For this review, take the finished solid that the model builds, in its own axes (mm). A direction names the side the tool comes from. Round coordinates to 2 decimals unless told otherwise and drop trailing zeros. Write each loop counter-clockwise with the first axis right and the second up, starting at its lowest first coordinate (ties: lowest second). Pieces come first, ordered by that corner, then holes. Notation, with made-up numbers: (7.5, 48) -> (51.5, 48) arc R8 ccw to (51.5, 53) -> close; hole circle Ø3 at (24.5, 17). An arc over 180 degrees is marked (long way). Write each question's results on one line, items separated by ' | '. Start each with the question number.
Item 1: Add section C-C (x = 33.65). State the section outline as (y, z) points, plus the area to 3 significant figures.
Item 2: Clearance check with flat-ended pins moving along their axes: pin 1 (8 mm diameter, centred on x = 13.25, y = -55.25, fed in from -Z); pin 2 (3 mm diameter, centred on y = -66, z = -5.5, fed in from +X); pin 3 (5 mm diameter, centred on x = 13, z = -3.5, fed in from +Y). State where each tip first meets the part, or that it passes through.
Item 3: Add section A-A (y = -38). State the section outline as (x, z) points, plus the area to 3 significant figures.
Item 4: Tool access review of faces 1 (the flat face through (11, -41, 1.2)), 2 (the cylindrical face through (-31.49, -19.65, 0.59)): name each direction out of +Z, -Z, +X, -X, +Y, -Y from which nothing blocks a thin tool from reaching the whole face with its end or side.
Item 5: Add section B-B (x = -39.75). State the section outline as (y, z) points.
Item 6: Add section D-D (z = -4.5). State the section outline as (x, y) points.
Item 7: The part is to be moulded in two halves that separate along X. For faces 3 (the cylindrical face through (-39.01, -43.17, 0.59)), 4 (the flat face through (14.5, -67, -5)), 5 (the flat face through (8.5, -67, -5)), say which applies: +X half, -X half, draft (parallel to the pull), parting line (faces both ways), or undercut.
Item 8: To check wall thickness, follow line 1 along Y through (x, z) = (-23.55, 0.7) (3 decimals); line 2 along Y through (x, z) = (2.75, 0.6); line 3 along X through (y, z) = (-58.5, 0.75). State the ranges of each line that lie inside material, in increasing order.
from build123d import *

# Parameters (mm, degrees)
SKETCH1_W                                    = 109.5
SKETCH1_H                                    = 82.5
SKETCH1_R                                    = 1.6
SKETCH1_R_2                                  = 1.05
SKETCH1_R_3                                  = 1.75
BOSS_EXTRUDE1_DEPTH                          = 1.2
CSK_FOR_M3_FLAT_COUNTERSUNK_HEAD_SCR_2_COUNT = 2
CSK_FOR_M3_FLAT_COUNTERSUNK_HEAD_SCR_2_PITCH = 76
CSK_FOR_M3_FLAT_COUNTERSUNK_HEAD_SCR_3_COUNT = 2
CSK_FOR_M3_FLAT_COUNTERSUNK_HEAD_SCR_3_PITCH = 122.834237898
CSK_FOR_M3_FLAT_COUNTERSUNK_HEAD_SCR_4_COUNT = 2
CSK_FOR_M3_FLAT_COUNTERSUNK_HEAD_SCR_4_PITCH = 96.5
F_2_6_2_6_DIAMETER_HOLE1_D                   = 2.6
CUT_EXTRUDE1_REACH                           = 101.438
SKETCH9_R                                    = 1.05
SKETCH9_R_2                                  = 3
SKETCH9_W                                    = 35
SKETCH9_H                                    = 46
SKETCH9_W_2                                  = 5.5
SKETCH9_H_2                                  = 13.4
FILLET1_R                                    = 3
FILLET2_R                                    = 1
SKETCH10_W                                   = 6
SKETCH10_H                                   = 6
BOSS_EXTRUDE2_DEPTH                          = 10


with BuildPart() as part:
    # Sketch1 → Boss-Extrude1 (new body)
    with BuildSketch(Plane.XY):
        with Locations((0, -41.75)):
            Rectangle(SKETCH1_W, SKETCH1_H)
        with Locations((-23.55, -67.625)):
            Circle(SKETCH1_R, mode=Mode.SUBTRACT)
        with Locations((-23.55, -15.875)):
            Circle(SKETCH1_R, mode=Mode.SUBTRACT)
        with Locations((-4.75, -6.75)):
            Circle(SKETCH1_R, mode=Mode.SUBTRACT)
        with Locations((-39.75, -41.75)):
            Circle(SKETCH1_R, mode=Mode.SUBTRACT)
        with Locations((19.998737342, -66.498737342)):
            Circle(SKETCH1_R, mode=Mode.SUBTRACT)
        with Locations((-12.25, -75.92862289)):
            Circle(SKETCH1_R_2, mode=Mode.SUBTRACT)
        with Locations((2.75, -75.92862289)):
            Circle(SKETCH1_R_2, mode=Mode.SUBTRACT)
        with Locations((26.542856399, -51.25)):
            Circle(SKETCH1_R_2, mode=Mode.SUBTRACT)
        with Locations((26.542856399, -32.25)):
            Circle(SKETCH1_R_2, mode=Mode.SUBTRACT)
        with Locations((39.65, -32.5)):
            Circle(SKETCH1_R_3, mode=Mode.SUBTRACT)
    extrude(amount=BOSS_EXTRUDE1_DEPTH)

    # Sketch3 → CSK for M3 Flat Countersunk Head Screw1 (revolve, cut)
    with BuildSketch(Plane(origin=(-48.25, -3.75, 1.2), x_dir=(0, -1, 0), z_dir=(1, 0, 0))):
        Polygon((0, 0), (0, 1.2), (1.6, 1.2), (1.6, 1.65), (3.25, 0), align=None)
    csk_for_m3_flat_countersunk_head_screw1 = revolve(axis=Axis((-48.25, -3.75, 7.55), (0, 0, -1)), mode=Mode.SUBTRACT)

    # CSK for M3 Flat Countersunk Head Scr 2: CSK for M3 Flat Countersunk Head Screw1 ×2
    with Locations(*[(0, -i * CSK_FOR_M3_FLAT_COUNTERSUNK_HEAD_SCR_2_PITCH, 0) for i in range(1, CSK_FOR_M3_FLAT_COUNTERSUNK_HEAD_SCR_2_COUNT)]):
        add(csk_for_m3_flat_countersunk_head_screw1, mode=Mode.SUBTRACT)

    # CSK for M3 Flat Countersunk Head Scr 3: CSK for M3 Flat Countersunk Head Screw1 ×2
    with Locations(*[Vector(0.7856115823348563, -0.6187200026678655, 0) * (i * CSK_FOR_M3_FLAT_COUNTERSUNK_HEAD_SCR_3_PITCH) for i in range(1, CSK_FOR_M3_FLAT_COUNTERSUNK_HEAD_SCR_3_COUNT)]):
        add(csk_for_m3_flat_countersunk_head_screw1, mode=Mode.SUBTRACT)

    # CSK for M3 Flat Countersunk Head Scr 4: CSK for M3 Flat Countersunk Head Screw1 ×2
    with Locations(*[(i * CSK_FOR_M3_FLAT_COUNTERSUNK_HEAD_SCR_4_PITCH, 0, 0) for i in range(1, CSK_FOR_M3_FLAT_COUNTERSUNK_HEAD_SCR_4_COUNT)]):
        add(csk_for_m3_flat_countersunk_head_screw1, mode=Mode.SUBTRACT)

    # Sketch5 → CSK for M2.5 Flat Countersunk Head Screw1 (revolve, cut)
    with BuildSketch(Plane(origin=(33.65, -11.85, 1.2), x_dir=(0, -1, 0), z_dir=(1, 0, 0))):
        Polygon((0, 0), (0, 1.2), (1.35, 1.2), (1.35, 1.5), (2.85, 0), align=None)
    revolve(axis=Axis((33.65, -11.85, 7.55), (0, 0, -1)), mode=Mode.SUBTRACT)

    # Ø2.6 (2.6) Diameter Hole1 (through all)
    with Locations(Plane.XY.offset(1.2)):
        with Locations((33.65, -2.32)):
            Hole(F_2_6_2_6_DIAMETER_HOLE1_D / 2)

    # Sketch9 → Cut-Extrude1 (cut, up to next)
    with BuildSketch(Plane.XY.offset(1.2), mode=Mode.PRIVATE) as cut_extrude1_sk1:
        with Locations((1.26040764, -13.467514421)):
            Circle(SKETCH9_R)
    cut_extrude1_tool1 = extrude(cut_extrude1_sk1.sketch, amount=-CUT_EXTRUDE1_REACH, mode=Mode.PRIVATE) & part.part
    # Sketch9 → Cut-Extrude1 (cut, up to next)
    with BuildSketch(Plane.XY.offset(1.2), mode=Mode.PRIVATE) as cut_extrude1_sk2:
        with Locations((6.91726189, -7.810660172)):
            Circle(SKETCH9_R)
    cut_extrude1_tool2 = extrude(cut_extrude1_sk2.sketch, amount=-CUT_EXTRUDE1_REACH, mode=Mode.PRIVATE) & part.part
    # Sketch9 → Cut-Extrude1 (cut, up to next)
    with BuildSketch(Plane.XY.offset(1.2), mode=Mode.PRIVATE) as cut_extrude1_sk3:
        with Locations((10.452795796, -11.346194078)):
            Circle(SKETCH9_R)
    cut_extrude1_tool3 = extrude(cut_extrude1_sk3.sketch, amount=-CUT_EXTRUDE1_REACH, mode=Mode.PRIVATE) & part.part
    # Sketch9 → Cut-Extrude1 (cut, up to next)
    with BuildSketch(Plane.XY.offset(1.2), mode=Mode.PRIVATE) as cut_extrude1_sk4:
        with Locations((13.25, -55.25)):
            Circle(SKETCH9_R_2)
    cut_extrude1_tool4 = extrude(cut_extrude1_sk4.sketch, amount=-CUT_EXTRUDE1_REACH, mode=Mode.PRIVATE) & part.part
    # Sketch9 → Cut-Extrude1 (cut, up to next)
    with BuildSketch(Plane.XY.offset(1.2), mode=Mode.PRIVATE) as cut_extrude1_sk5:
        with Locations((4.795941546, -17.003048327)):
            Circle(SKETCH9_R)
    cut_extrude1_tool5 = extrude(cut_extrude1_sk5.sketch, amount=-CUT_EXTRUDE1_REACH, mode=Mode.PRIVATE) & part.part
    # Sketch9 → Cut-Extrude1 (cut, up to next)
    with BuildSketch(Plane.XY.offset(1.2), mode=Mode.PRIVATE) as cut_extrude1_sk6:
        with Locations((11.867009358, -18.41726189)):
            Circle(SKETCH9_R)
    cut_extrude1_tool6 = extrude(cut_extrude1_sk6.sketch, amount=-CUT_EXTRUDE1_REACH, mode=Mode.PRIVATE) & part.part
    # Sketch9 → Cut-Extrude1 (cut, up to next)
    with BuildSketch(Plane.XY.offset(1.2), mode=Mode.PRIVATE) as cut_extrude1_sk7:
        with Locations((-14.85, -41.75)):
            Rectangle(SKETCH9_W, SKETCH9_H)
    cut_extrude1_tool7 = extrude(cut_extrude1_sk7.sketch, amount=-CUT_EXTRUDE1_REACH, mode=Mode.PRIVATE) & part.part
    # Sketch9 → Cut-Extrude1 (cut, up to next)
    with BuildSketch(Plane.XY.offset(1.2), mode=Mode.PRIVATE) as cut_extrude1_sk8:
        with BuildLine():
            Line((7.624368671, -15.588834765), (-2.982233047, -4.982233047))
            ThreePointArc((-2.982233047, -4.982233047), (-2.982233047, -3.568019485), (-1.568019485, -3.568019485))
            Line((-1.568019485, -3.568019485), (9.038582233, -14.174621202))
            ThreePointArc((9.038582233, -14.174621202), (9.038582233, -15.588834765), (7.624368671, -15.588834765))
        make_face()
    cut_extrude1_tool8 = extrude(cut_extrude1_sk8.sketch, amount=-CUT_EXTRUDE1_REACH, mode=Mode.PRIVATE) & part.part
    # Sketch9 → Cut-Extrude1 (cut, up to next)
    with BuildSketch(Plane.XY.offset(1.2), mode=Mode.PRIVATE) as cut_extrude1_sk9:
        with Locations((46.25, -41.75)):
            Rectangle(SKETCH9_W_2, SKETCH9_H_2)
    cut_extrude1_tool9 = extrude(cut_extrude1_sk9.sketch, amount=-CUT_EXTRUDE1_REACH, mode=Mode.PRIVATE) & part.part
    add(cut_extrude1_tool1.solids().sort_by_distance((1.260408, -13.467514, 1.2))[0], mode=Mode.SUBTRACT)
    add(cut_extrude1_tool2.solids().sort_by_distance((6.917262, -7.81066, 1.2))[0], mode=Mode.SUBTRACT)
    add(cut_extrude1_tool3.solids().sort_by_distance((10.452796, -11.346194, 1.2))[0], mode=Mode.SUBTRACT)
    add(cut_extrude1_tool4.solids().sort_by_distance((13.25, -55.25, 1.2))[0], mode=Mode.SUBTRACT)
    add(cut_extrude1_tool5.solids().sort_by_distance((4.795942, -17.003048, 1.2))[0], mode=Mode.SUBTRACT)
    add(cut_extrude1_tool6.solids().sort_by_distance((11.867009, -18.417262, 1.2))[0], mode=Mode.SUBTRACT)
    add(cut_extrude1_tool7.solids().sort_by_distance((-14.85, -41.75, 1.2))[0], mode=Mode.SUBTRACT)
    add(cut_extrude1_tool8.solids().sort_by_distance((3.028175, -9.578427, 1.2))[0], mode=Mode.SUBTRACT)
    add(cut_extrude1_tool9.solids().sort_by_distance((46.25, -41.75, 1.2))[0], mode=Mode.SUBTRACT)

    # Fillet1
    fillet1_edges = [part.edges().sort_by_distance(p)[0] for p in [
        (2.65, -18.75, 0.6),
        (2.65, -64.75, 0.6),
        (-32.35, -64.75, 0.6),
        (-32.35, -18.75, 0.6),
    ]]
    fillet(fillet1_edges, radius=FILLET1_R)

    # Fillet2
    fillet2_edges = [part.edges().sort_by_distance(p)[0] for p in [
        (43.5, -48.45, 0.6),
        (43.5, -35.05, 0.6),
        (49, -35.05, 0.6),
        (49, -48.45, 0.6),
    ]]
    fillet(fillet2_edges, radius=FILLET2_R)

    # Sketch10 → Boss-Extrude2 (add)
    with BuildSketch(Plane(origin=(0, 0, 0), x_dir=(-1, 0, 0), z_dir=(0, 0, -1))):
        with Locations((-11.5, -67)):
            Rectangle(SKETCH10_W, SKETCH10_H)
    extrude(amount=BOSS_EXTRUDE2_DEPTH)


solid = part.part
Responses:
1) outline: (-83, 0) -> (-13.5, 0) -> (-14.7, 1.2) -> (-83, 1.2) -> close; (-10.2, 0) -> (-3.62, 0) -> (-3.62, 1.2) -> (-9, 1.2) -> close; (-1.02, 0) -> (-0.5, 0) -> (-0.5, 1.2) -> (-1.02, 1.2) -> close | area: 90.5 mm^2
2) pin 1: stops at z = 0 | pin 2: stops at x = 14.5 | pin 3: stops at y = -64
3) outline: (-54.75, 0) -> (-32.35, 0) -> (-32.35, 1.2) -> (-54.75, 1.2) -> close; (2.65, 0) -> (43.5, 0) -> (43.5, 1.2) -> (2.65, 1.2) -> close; (49, 0) -> (54.75, 0) -> (54.75, 1.2) -> (49, 1.2) -> close | area: 82.8 mm^2
4) face 1: +Z, +X, -X, +Y, -Y | face 2: +Z, -Z
5) outline: (-83, 0) -> (-43.35, 0) -> (-43.35, 1.2) -> (-83, 1.2) -> close; (-40.15, 0) -> (-0.5, 0) -> (-0.5, 1.2) -> (-40.15, 1.2) -> close
6) outline: (8.5, -70) -> (14.5, -70) -> (14.5, -64) -> (8.5, -64) -> close
7) face 3: undercut | face 4: +X half | face 5: -X half
8) line 1: y = -83 to -69.225, -66.025 to -64.75, -18.75 to -17.475, -14.275 to -0.5 | line 2: y = -83 to -76.98, -74.88 to -10.71, -7.89 to -0.5 | line 3: x = -54.75 to -32.35, 2.65 to 54.75
